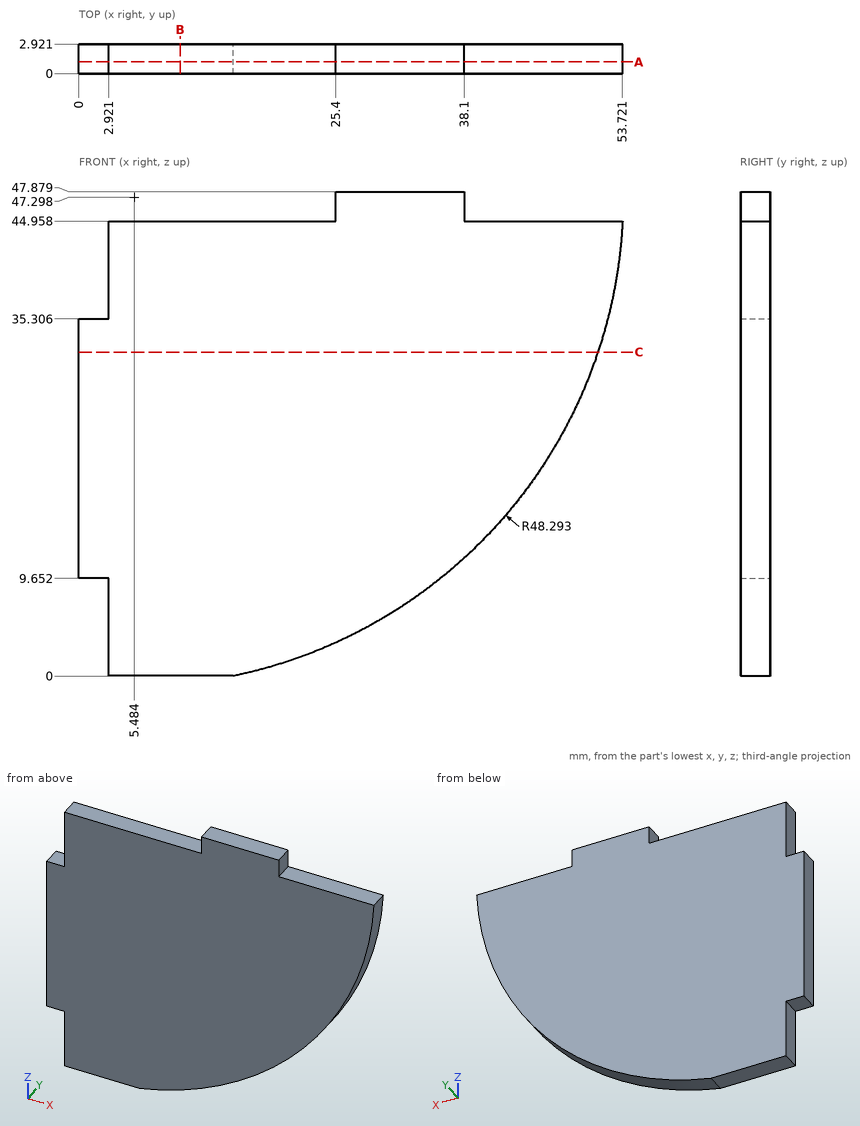
Check sheet for the drawn part. Datum: minimum x, y, z corner. Units: mm. Give positions to 0.01 mm unless a question says otherwise; leave off trailing zeros. Loops run counter-clockwise (first coordinate to the right, second up) from the corner with the lowest first, then second, coordinate; pieces in that order, holes last. Notation, with made-up numbers: (39, -38) - (73, -38) arc R27 cw to (73, -5) - close; hole circle Ø11 at (20.5, -8). An arc over 180 degrees is marked (long way). Write each question's results on one line, items separated by ' | '.
1) Sectioned sample at C-C on z = 32. Record the boundary of the cut face in (x, y), plus the area to 3 significant figures.
Solution:
outline: (0, 0) - (51.29, 0) - (51.29, 2.92) - (0, 2.92) - close | area: 150 mm2
2) Depth check by flat-ended pin: P1, Ø1.5, axis at y = 1.5, z = 5, coming from the -X side; P2, Ø0.9, axis at y = 2, z = 46, coming from the +X side; P3, Ø1.5, axis at x = 1, y = 1.5, coming from the -Z side. Enter the tip coordinate at first touch or a pass-through.
Solution:
P1: x = 2.92 | P2: x = 38.1 | P3: z = 9.65
3) Sectioned sample at A-A on y = 1.15. Record the boundary of the cut face in (x, z) (1 decimal), plus the area to 3 significant figures.
Solution:
outline: (0, 9.7) - (2.9, 9.7) - (2.9, 0) - (15.2, 0) arc R48.3 ccw to (53.7, 45) - (38.1, 45) - (38.1, 47.9) - (25.4, 47.9) - (25.4, 45) - (2.9, 45) - (2.9, 35.3) - (0, 35.3) - close | area: 1,940 mm2
4) Sectioned sample at B-B on x = 10. Record the boundary of the cut face in (y, z), plus the area to 3 significant figures.
Solution:
outline: (0, 0) - (2.92, 0) - (2.92, 44.96) - (0, 44.96) - close | area: 131 mm2
5) Material ranges on L1, parallel to Z at x = 13.5, y = 2.6; L2, parallel to X at y = 1.4, z = 45.5; L3, parallel to X at y = 2, z = 33, recorded low to high. Write a range as from..to.
Solution:
L1: 0..44.96 | L2: 25.4..38.1 | L3: 0..51.61
